Autodesk Inventor part; units mm, degrees
ref_plane "YZ Plane" through (0, 0, 0) normal (1, 0, 0) x (0, 1, 0)
ref_plane "XZ Plane" through (0, 0, 0) normal (0, 1, 0) x (-1, 0, 0)
ref_plane "XY Plane" through (0, 0, 0) normal (0, 0, 1) x (1, 0, 0)
sketch "Sketch1" plane through (0, 0, 0) normal (0, 1, 0) x (-1, 0, 0)
  line L0 (0, 0) -> (44, 0)
  line L1 (44, -75) -> (20, -75)
  line L2 (0, -75) -> (0, -7)
  line L3 (44, 0) -> (44, -7)
  line L4 (44, -7) -> (34, -7)
  line L5 (34, -7) -> (34, -68)
  line L6 (34, -68) -> (44, -68)
  line L7 (44, 0) -> (44, -7)
  line L8 (44, -68) -> (44, -75)
  line L9 (0, 0) -> (20, 0)
  line L10 (20, 0) -> (20, -7)
  line L11 (20, -7) -> (0, -7)
  line L12 (20, -68) -> (20, -75)
  line L13 (20, -68) -> (0, -68)
  dimension "d0" = 44
  dimension "d1" = 75
  dimension "d2" = 7
  dimension "d3" = 10
  dimension "d4" = 61
  dimension "d5" = 20
extrude "Extrusion1" add sketch "Sketch1" along normal blind 1
sketch "Sketch2" plane through (0, 1, 0) normal (0, 1, 0) x (1, 0, 0)
  line L0 (0, 68) -> (-20, 68)
  line L1 (-20, 75) -> (-44, 75)
  line L2 (-34, 7) -> (-44, 7)
  line L3 (-44, 0) -> (-43, 0)
  line L4 (-43, 0) -> (-43, 7)
  line L5 (-43, 7) -> (-44, 7)
  line L6 (-44, 7) -> (-44, 0)
  line L7 (-44, 68) -> (-43, 68)
  line L8 (-43, 68) -> (-43, 75)
  line L9 (-43, 75) -> (-44, 75)
  line L10 (-44, 75) -> (-44, 68)
  line L11 (0, 7) -> (-1, 7)
  line L12 (-1, 7) -> (-1, 68)
  line L13 (-1, 68) -> (0, 68)
  line L14 (0, 68) -> (0, 7)
  point P0 (0, 0)
  dimension "d8" = 1
  dimension "d9" = 1
  dimension "d10" = 1
extrude "Extrusion2" add sketch "Sketch2" along normal blind 30
sketch "Sketch3" plane through (-44, 0, -7) normal (-1, 0, 0) x (0, 0, 1)
  line L0 (0, 31) -> (7, 31)
  line L1 (3.5, 31) -> (3.5, 25)
  line L2 (3.5, 25) -> (3.5, 9)
  circle A0 centre (3.5, 25) radius 2
  circle A1 centre (3.5, 9) radius 2
  dimension "d13" = 6
  dimension "d14" = 16
  dimension "d15" = 4
  dimension "d16" = 4
extrude "Extrusion3" cut sketch "Sketch3" against normal blind 30
sketch "Sketch4" plane through (-44, 0, -75) normal (-1, 0, 0) x (0, 0, 1)
  line L0 (7, 31) -> (0, 31)
  line L1 (3.5, 31) -> (3.5, 25)
  line L2 (3.5, 25) -> (3.5, 9)
  circle A0 centre (3.5, 25) radius 2
  circle A1 centre (3.5, 9) radius 2
  point P0 (75, 0)
  dimension "d19" = 6
  dimension "d20" = 16
  dimension "d21" = 4
  dimension "d22" = 4
extrude "Extrusion4" cut sketch "Sketch4" against normal blind 30
properties part number "Shoulder Plate"
Geometry check sheet. Reference: the model listing, model coordinates, mm. A direction names the side the tool comes from. Round coordinates to 2 decimals unless told otherwise and drop trailing zeros. Loops run counter-clockwise (first coordinate to the right, second up) from the corner with the lowest first, then second, coordinate; pieces in that order, holes last. Notation, with made-up numbers: (-7.75, 45) - (30.25, 45) arc R31 ccw to (30.25, 77) - close; hole circle Ø6 at (40, -38.75). An arc over 180 degrees is marked (long way). Write each question's results on one line, items separated by ' | '. Start each with the question number.
Q1. Cross-section at D-D on y = 6. Enter the section's corners in (x, z).
Q2. Access from +Z, -Z, +X, -X, +Y, -Y to the whole of each face (thin tool, end or side, straight path). Record for faces 5 (the flat face through (-43, 16, -3)), 6 (the flat face through (-1, 16, -37)), 7 (the flat face through (-0.4, 8.5, -68)), 8 (the flat face through (-0.4, 8.5, -7)), 9 (the flat face through (-43.4, 12, -68)).
Q3. Cross-section at A-A on y = 25. Enter the section's corners in (x, z).
Q4. Cross-section at C-C on x = -37. Enter the section's corners in (y, z).
Q5. Gauge pin test, flat ends, axial feed: P1, Ø8, axis at x = -28, z = -34.5, coming from the -Y side; P2, Ø5, axis at x = -33.5, z = -13, coming from the +Y side; P3, Ø9, axis at y = 21, z = -31, coming from the -X side; P4, Ø5, axis at y = 9, z = -71.5, coming from the +X side. Record the tip position at first contact, or that the pin passes through.
Q6. Release check for a two-part mould opening along Y. For faces 1 (the cylindrical face through (-43.507, 10.983, -3.76)), 2 (the flat face through (-22, 0, -37)), 3 (the flat face through (-43, 16, -71)), 4 (the flat face through (-22, 1, -37)) record: +Y half, -Y half, draft (parallel to the pull), parting line (faces both ways), or undercut.
Q7. Cross-section at B-B on z = -71.5. Enter the section's corners in (x, y).
Q8. Thickness scan on line 1 (Y direction, x = -43.5, z = -3.5); line 2 (Z direction, x = -43.6, y = 25); line 3 (X direction, y = 24, z = -46). Record the ranges inside material, lowest first. Write a range as [from, to].
Answers below:
1) outline: (-44, -75) - (-43, -75) - (-43, -68) - (-44, -68) - close; (-44, -7) - (-43, -7) - (-43, 0) - (-44, 0) - close; (-1, -68) - (0, -68) - (0, -7) - (-1, -7) - close
2) face 5: +Z, -Z, +X, +Y | face 6: +Z, -Z, -X, +Y | face 7: -Z, +X, +Y, -Y | face 8: +Z, +X, +Y, -Y | face 9: -X, +Y, -Y
3) outline: (-44, -75) - (-43, -75) - (-43, -73.5) - (-44, -73.5) - close; (-44, -69.5) - (-43, -69.5) - (-43, -68) - (-44, -68) - close; (-44, -7) - (-43, -7) - (-43, -5.5) - (-44, -5.5) - close; (-44, -1.5) - (-43, -1.5) - (-43, 0) - (-44, 0) - close; (-1, -68) - (0, -68) - (0, -7) - (-1, -7) - close
4) outline: (0, -75) - (1, -75) - (1, -68) - (0, -68) - close; (0, -7) - (1, -7) - (1, 0) - (0, 0) - close
5) P1: stops at y = 0 | P2: stops at y = 1 | P3: stops at x = -1 | P4: stops at x = -43
6) face 1: undercut | face 2: -Y half | face 3: draft | face 4: +Y half
7) outline: (-44, 0) - (-20, 0) - (-20, 1) - (-43, 1) - (-43, 7) - (-44, 7) - close; (-44, 11) - (-43, 11) - (-43, 23) - (-44, 23) - close; (-44, 27) - (-43, 27) - (-43, 31) - (-44, 31) - close
8) line 1: y = [0, 7], [11, 23], [27, 31] | line 2: z = [-75, -73.5], [-69.5, -68], [-7, -5.5], [-1.5, 0] | line 3: x = [-1, 0]
